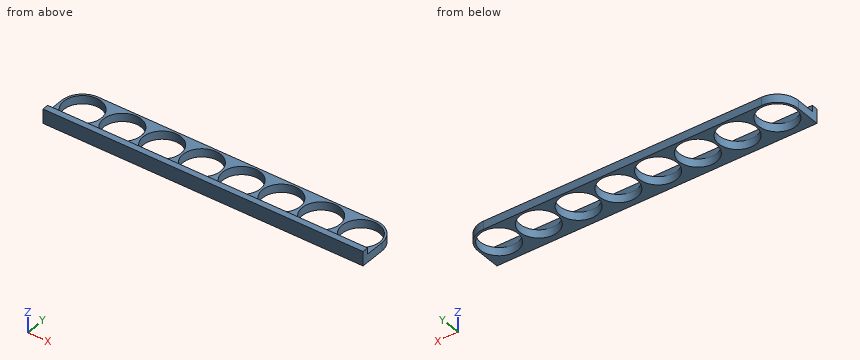
from build123d import *

# Parameters (mm, degrees)
SKETCH1_R           = 9.2
BOSS_EXTRUDE1_DEPTH = 4
SKETCH2_W           = 156.2
SKETCH2_H           = 3
BOSS_EXTRUDE2_DEPTH = 3


with BuildPart() as part:
    # Sketch1 → Boss-Extrude1 (new body)
    with BuildSketch(Plane.XY):
        with BuildLine():
            Line((0, 10.2), (135.8, 10.2))
            ThreePointArc((135.8, 10.2), (143.012489168, 7.212489168), (146, 0))
            Line((146, 0), (146, -12.2))
            Line((146, -12.2), (-10.2, -12.2))
            Line((-10.2, -12.2), (-10.2, 0))
            ThreePointArc((-10.2, 0), (-7.212489168, 7.212489168), (0, 10.2))
        make_face()
        Circle(SKETCH1_R, mode=Mode.SUBTRACT)
        with Locations((19.4, 0)):
            Circle(SKETCH1_R, mode=Mode.SUBTRACT)
        with Locations((38.8, 0)):
            Circle(SKETCH1_R, mode=Mode.SUBTRACT)
        with Locations((58.2, 0)):
            Circle(SKETCH1_R, mode=Mode.SUBTRACT)
        with Locations((77.6, 0)):
            Circle(SKETCH1_R, mode=Mode.SUBTRACT)
        with Locations((97, 0)):
            Circle(SKETCH1_R, mode=Mode.SUBTRACT)
        with Locations((116.4, 0)):
            Circle(SKETCH1_R, mode=Mode.SUBTRACT)
        with Locations((135.8, 0)):
            Circle(SKETCH1_R, mode=Mode.SUBTRACT)
    extrude(amount=BOSS_EXTRUDE1_DEPTH)

    # Sketch2 → Boss-Extrude2 (add)
    with BuildSketch(Plane.XY.offset(4)):
        with Locations((67.9, -10.7)):
            Rectangle(SKETCH2_W, SKETCH2_H)
    extrude(amount=BOSS_EXTRUDE2_DEPTH)


solid = part.part
Model file for the job. Use its own axes, mm. Give positions to 0.01 mm unless a question says otherwise; leave off trailing zeros. Write each loop counter-clockwise with the first axis right and the second up, starting at its lowest first coordinate (ties: lowest second). Pieces come first, ordered by that corner, then holes. Notation, with made-up numbers: (67.25, 12) -> (72.25, 12) arc R28 ccw to (72.25, 35) -> close; hole circle Ø11 at (8.25, -11.75). An arc over 180 degrees is marked (long way). Write item = value, one per line.
(1) Slice it at A-A, the plane z = 1.75. Give the number of separate pieces and of enclosed holes in the cut face, then the cut area to 3 significant figures.
Determined:
separate_pieces = 1
enclosed_holes = 8
area = 1,330 mm2
(2) Probe line 1 along Y through (x, z) = (38.8, 1.15); line 2 along Y through (x, z) = (29, 6.5); line 3 along Z through (x, y) = (44.5, 8.5). List the from-to ranges inside material, lowest first.
Determined:
line_1 = -12.2 to -9.2, 9.2 to 10.2
line_2 = -12.2 to -9.2
line_3 = 0 to 4
(3) Slice it at D-D, the plane x = 32. Give the cut face in (y, z).
Determined:
outline = (-12.2, 0) -> (-6.2, 0) -> (-6.2, 4) -> (-9.2, 4) -> (-9.2, 7) -> (-12.2, 7) -> close; (6.2, 0) -> (10.2, 0) -> (10.2, 4) -> (6.2, 4) -> close
(4) Flat gauge pins, fed straight in: P1, Ø10, axis at x = 24.5, y = 0, coming from the +Z side; P2, Ø3.5, axis at x = 37.5, z = 6, coming from the +Y side; P3, Ø4, axis at x = 51.5, y = -2, coming from the +Z side. Where does each tip first touch, or does it go through?
Determined:
P1 = 4
P2 = -9.2
P3 = through
(5) Slice it at B-B, the plane x = 85. Give the cut face in (y, z), then the cut area to 3 significant figures.
Determined:
outline = (-12.2, 0) -> (-5.47, 0) -> (-5.47, 4) -> (-9.2, 4) -> (-9.2, 7) -> (-12.2, 7) -> close; (5.47, 0) -> (10.2, 0) -> (10.2, 4) -> (5.47, 4) -> close
area = 54.9 mm2
